Verification items for the finished model (mm, model axes). Face numbers are marked on the shaded views. A direction names the side the tool comes from. Give positions to 0.01 mm unless a question says otherwise; leave off trailing zeros. Order: outer loops, then holes, each group sorted by start corner. A loop starts at its lowest first (then second) coordinate and runs counter-clockwise, first axis right, second up.
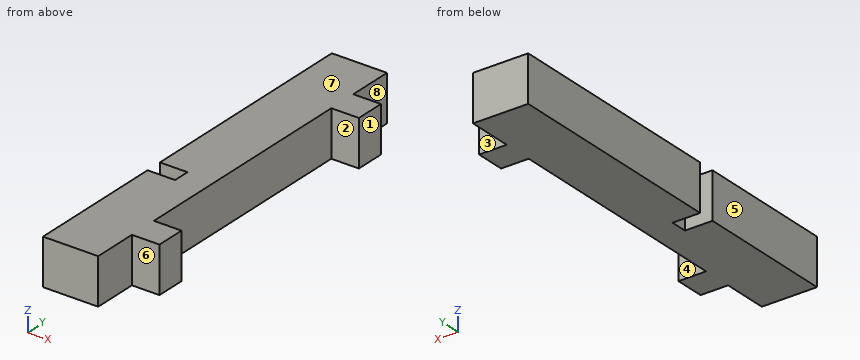
Autodesk Inventor part; units mm, degrees
ref_plane "YZ Plane" through (0, 0, 0) normal (1, 0, 0) x (0, 1, 0)
ref_plane "XZ Plane" through (0, 0, 0) normal (0, 1, 0) x (-1, 0, 0)
ref_plane "XY Plane" through (0, 0, 0) normal (0, 0, 1) x (1, 0, 0)
sketch "Sketch1" plane through (0, 0, 0) normal (0, 0, 1) x (1, 0, 0)
  line L0 (0, 42) -> (6, 42)
  line L1 (6, 42) -> (6, 0)
  line L2 (6, 0) -> (0, 0)
  line L3 (0, 0) -> (0, 42)
  dimension "d0" = 6
  dimension "d1" = 42
extrude "Extrusion1" add sketch "Sketch1" against normal blind 5
sketch "Sketch4" plane through (0, 0, 0) normal (0, 0, 1) x (1, 0, 0)
  line L0 (0, 0) -> (0, 42)
  line L1 (0, 17) -> (3, 17)
  line L2 (3, 17) -> (3, 15.2)
  line L3 (3, 15.2) -> (0, 15.2)
  line L4 (0, 15.2) -> (0, 17)
  line L5 (6, 0) -> (0, 0)
  point P0 (0, 45)
  dimension "d12" = 1.8
  dimension "d13" = 3
  dimension "d18" = 17
extrude "Extrusion4" cut sketch "Sketch4" against normal blind 5
sketch "Sketch5" plane through (0, 0, 0) normal (0, 0, 1) x (1, 0, 0)
  line L0 (6, 42) -> (6, 0)
  line L1 (6, 0) -> (0, 0)
  line L2 (0, 42) -> (6, 42)
  line L3 (6, 42) -> (6, 0)
  line L4 (9, 8.1) -> (6, 8.1)
  line L5 (6, 8.1) -> (6, 4.9)
  line L6 (6, 4.9) -> (9, 4.9)
  line L7 (9, 4.9) -> (9, 8.1)
  line L8 (9, 8.1) -> (6, 4.9) construction
  line L9 (6, 8.1) -> (9, 4.9) construction
  line L10 (9, 37.1) -> (6, 37.1)
  line L11 (6, 37.1) -> (6, 33.9)
  line L12 (6, 33.9) -> (9, 33.9)
  line L13 (9, 33.9) -> (9, 37.1)
  line L14 (9, 37.1) -> (6, 33.9) construction
  line L15 (6, 37.1) -> (9, 33.9) construction
  line L16 (0, 42) -> (6, 0) construction
  line L17 (0, 0) -> (6, 42) construction
  point P0 (7.5, 6.5)
  point P1 (7.5, 35.5)
  point P2 (3, 21)
  dimension "d31" = 3
  dimension "d32" = 3.2
  dimension "d34" = 14.5
  dimension "d35" = 14.5
  dimension "d36" = 3.2
extrude "Extrusion5" add sketch "Sketch5" against normal blind 5
equation "\"d36\" = d32"
equation "\"kerf\" = 0.15"
properties part number "PCBSupport"
(1) Go/stop test with flat-tipped pins: pin 1 (1.5 mm diameter, centred on x = 7, z = -1.5, fed in from +Y); pin 2 (2.5 mm diameter, centred on y = 1.5, z = -3.5, fed in from +X); pin 3 (0.9 mm diameter, centred on y = 16, z = -2, fed in from -X). Record where each tip stops, or that it passes through.
Solved:
pin 1: stops at y = 37.1
pin 2: stops at x = 6
pin 3: stops at x = 3
(2) Scan lines: line 1 (Y direction, x = 2.5, z = -0.3); line 2 (Y direction, x = 8.25, z = -2.2); line 3 (X direction, y = 31.5, z = -4.6). Record each from-to range of solid material in increasing order.
Solved:
line 1: y = 0 to 15.2, 17 to 42
line 2: y = 4.9 to 8.1, 33.9 to 37.1
line 3: x = 0 to 6
(3) Section check C-C, the plane y = 19. Enter the section's corners in (x, z), then the cut area to 3 significant figures.
Solved:
outline: (0, -5) - (6, -5) - (6, 0) - (0, 0) - close
area: 30.0 mm2
(4) Set-up check for the marked faces 4, 5, 6, 7 and 8: record each of +Z, -Z, +X, -X, +Y, -Y from which the full face is reachable in a straight line by a thin tool's end or side.
Solved:
face 4: +Z, -Z, +X
face 5: +Z, -Z, -X, +Y, -Y
face 6: +Z, -Z, +X, -Y
face 7: +Z, +X, -X, +Y, -Y
face 8: +Z, -Z, +X, +Y
(5) Section check D-D, the plane x = 0.5. Enter the section's corners in (y, z).
Solved:
outline: (0, -5) - (15.2, -5) - (15.2, 0) - (0, 0) - close; (17, -5) - (42, -5) - (42, 0) - (17, 0) - close
(6) Release check for a two-part mould opening along Y. For the marked faces 1, 2 and 3 record: pulls with the +Y half, pulls with the -Y half, needs draft (parallel to the pull), parting line crosses it, or undercut.
Solved:
face 1: needs draft
face 2: undercut
face 3: pulls with the +Y half
(7) Section check A-A, the plane x = 7.75. Enter the section's corners in (y, z).
Solved:
outline: (4.9, -5) - (8.1, -5) - (8.1, 0) - (4.9, 0) - close; (33.9, -5) - (37.1, -5) - (37.1, 0) - (33.9, 0) - close
(8) Section check B-B, the plane z = -2.5. Enter the section's corners in (x, y).
Solved:
outline: (0, 0) - (6, 0) - (6, 4.9) - (9, 4.9) - (9, 8.1) - (6, 8.1) - (6, 33.9) - (9, 33.9) - (9, 37.1) - (6, 37.1) - (6, 42) - (0, 42) - (0, 17) - (3, 17) - (3, 15.2) - (0, 15.2) - close
